Input: part model. Units: mm. Frame: model coordinates. Coordinates: 2 decimals unless noted, no trailing zeros. Loops run counter-clockwise (first coordinate to the right, second up) from the corner with the lowest first, then second, coordinate; pieces in that order, holes last.
Item 1: Section A-A on y = 128. Return loops of the section in (x, z), and give its area (3 significant figures).
Item 2: Ray query, line 1 along X through (y, z) = (164, -1.4); line 2 along Y through (x, z) = (-80, 0.85) (3 decimals); line 3 along Y through (x, z) = (14.5, -0.75) (3 decimals). Return the intervals inside material, ascending.
Item 3: Section C-C on z = -0.1. Give the number of separate pieces and of enclosed holes in the cut face, and give its area (3 significant figures).
```python
from build123d import *

# Parameters (mm, degrees)
SKETCH1_W                     = 382.775
SKETCH1_H                     = 238.275
BOSS_EXTRUDE1_DEPTH           = 1.5875
SKETCH3_W                     = 38.1
SKETCH3_H                     = 6.35
WELD_TABS_EXTRUDE_DEPTH       = 3.175
SKETCH4_R                     = 1.5875
WELD_TABS_TEAR_DROP_CUT_DEPTH = 3.175
WELD_TABS_CUTOUT_DEPTH        = 3.175


with BuildPart() as part:
    # Sketch1 → Boss-Extrude1 (new body, symmetric)
    with BuildSketch(Plane.XY):
        with Locations((-158.05, 122.3125)):
            Rectangle(SKETCH1_W, SKETCH1_H)
    extrude(amount=BOSS_EXTRUDE1_DEPTH, both=True)

    # Sketch3 → Weld Tabs Extrude (add)
    with BuildSketch(Plane.XY.offset(1.5875)):
        with Locations((-237.075, 0)):
            Rectangle(SKETCH3_W, SKETCH3_H)
        with Locations((-158.05, 0)):
            Rectangle(SKETCH3_W, SKETCH3_H)
        with Locations((-79.025, 0)):
            Rectangle(SKETCH3_W, SKETCH3_H)
    extrude(amount=-WELD_TABS_EXTRUDE_DEPTH)

    # Sketch4 → Weld Tabs Tear Drop Cut (cut)
    with BuildSketch(Plane.XY.offset(1.5875)):
        with Locations((-257.247532015, 2.052467985)):
            Circle(SKETCH4_R)
        with Locations((-216.902467985, 2.052467985)):
            Circle(SKETCH4_R)
        with Locations((-178.222532015, 2.052467985)):
            Circle(SKETCH4_R)
        with Locations((-137.877467985, 2.052467985)):
            Circle(SKETCH4_R)
        with Locations((-99.197532015, 2.052467985)):
            Circle(SKETCH4_R)
        with Locations((-58.852467985, 2.052467985)):
            Circle(SKETCH4_R)
    extrude(amount=-WELD_TABS_TEAR_DROP_CUT_DEPTH, mode=Mode.SUBTRACT)

    # Sketch6 → Weld Tabs Cutout (cut)
    with BuildSketch(Plane.XY.offset(1.5875)):
        with BuildLine():
            Line((-238.6625, 200.93125), (-238.6625, 162.83125))
            ThreePointArc((-238.6625, 162.83125), (-237.075, 161.24375), (-235.4875, 162.83125))
            Line((-235.4875, 162.83125), (-235.4875, 200.93125))
            ThreePointArc((-235.4875, 200.93125), (-237.075, 202.51875), (-238.6625, 200.93125))
        make_face()
        with BuildLine():
            Line((-317.6875, 200.93125), (-317.6875, 162.83125))
            ThreePointArc((-317.6875, 162.83125), (-316.1, 161.24375), (-314.5125, 162.83125))
            Line((-314.5125, 162.83125), (-314.5125, 200.93125))
            ThreePointArc((-314.5125, 200.93125), (-316.1, 202.51875), (-317.6875, 200.93125))
        make_face()
        with BuildLine():
            Line((-159.6375, 200.93125), (-159.6375, 162.83125))
            ThreePointArc((-159.6375, 162.83125), (-158.05, 161.24375), (-156.4625, 162.83125))
            Line((-156.4625, 162.83125), (-156.4625, 200.93125))
            ThreePointArc((-156.4625, 200.93125), (-158.05, 202.51875), (-159.6375, 200.93125))
        make_face()
        with BuildLine():
            Line((-80.6125, 200.93125), (-80.6125, 162.83125))
            ThreePointArc((-80.6125, 162.83125), (-79.025, 161.24375), (-77.4375, 162.83125))
            Line((-77.4375, 162.83125), (-77.4375, 200.93125))
            ThreePointArc((-77.4375, 200.93125), (-79.025, 202.51875), (-80.6125, 200.93125))
        make_face()
        with BuildLine():
            Line((-1.5875, 200.93125), (-1.5875, 162.83125))
            ThreePointArc((-1.5875, 162.83125), (0, 161.24375), (1.5875, 162.83125))
            Line((1.5875, 162.83125), (1.5875, 200.93125))
            ThreePointArc((1.5875, 200.93125), (0, 202.51875), (-1.5875, 200.93125))
        make_face()
        with BuildLine():
            Line((-238.6625, 141.3625), (-238.6625, 103.2625))
            ThreePointArc((-238.6625, 103.2625), (-237.075, 101.675), (-235.4875, 103.2625))
            Line((-235.4875, 103.2625), (-235.4875, 141.3625))
            ThreePointArc((-235.4875, 141.3625), (-237.075, 142.95), (-238.6625, 141.3625))
        make_face()
        with BuildLine():
            Line((-159.6375, 141.3625), (-159.6375, 103.2625))
            ThreePointArc((-159.6375, 103.2625), (-158.05, 101.675), (-156.4625, 103.2625))
            Line((-156.4625, 103.2625), (-156.4625, 141.3625))
            ThreePointArc((-156.4625, 141.3625), (-158.05, 142.95), (-159.6375, 141.3625))
        make_face()
        with BuildLine():
            Line((-80.6125, 141.3625), (-80.6125, 103.2625))
            ThreePointArc((-80.6125, 103.2625), (-79.025, 101.675), (-77.4375, 103.2625))
            Line((-77.4375, 103.2625), (-77.4375, 141.3625))
            ThreePointArc((-77.4375, 141.3625), (-79.025, 142.95), (-80.6125, 141.3625))
        make_face()
        with BuildLine():
            Line((-1.5875, 141.3625), (-1.5875, 103.2625))
            ThreePointArc((-1.5875, 103.2625), (0, 101.675), (1.5875, 103.2625))
            Line((1.5875, 103.2625), (1.5875, 141.3625))
            ThreePointArc((1.5875, 141.3625), (0, 142.95), (-1.5875, 141.3625))
        make_face()
        with BuildLine():
            Line((-238.6625, 81.79375), (-238.6625, 43.69375))
            ThreePointArc((-238.6625, 43.69375), (-237.075, 42.10625), (-235.4875, 43.69375))
            Line((-235.4875, 43.69375), (-235.4875, 81.79375))
            ThreePointArc((-235.4875, 81.79375), (-237.075, 83.38125), (-238.6625, 81.79375))
        make_face()
        with BuildLine():
            Line((-159.6375, 81.79375), (-159.6375, 43.69375))
            ThreePointArc((-159.6375, 43.69375), (-158.05, 42.10625), (-156.4625, 43.69375))
            Line((-156.4625, 43.69375), (-156.4625, 81.79375))
            ThreePointArc((-156.4625, 81.79375), (-158.05, 83.38125), (-159.6375, 81.79375))
        make_face()
        with BuildLine():
            Line((-80.6125, 81.79375), (-80.6125, 43.69375))
            ThreePointArc((-80.6125, 43.69375), (-79.025, 42.10625), (-77.4375, 43.69375))
            Line((-77.4375, 43.69375), (-77.4375, 81.79375))
            ThreePointArc((-77.4375, 81.79375), (-79.025, 83.38125), (-80.6125, 81.79375))
        make_face()
        with BuildLine():
            Line((-1.5875, 81.79375), (-1.5875, 43.69375))
            ThreePointArc((-1.5875, 43.69375), (0, 42.10625), (1.5875, 43.69375))
            Line((1.5875, 43.69375), (1.5875, 81.79375))
            ThreePointArc((1.5875, 81.79375), (0, 83.38125), (-1.5875, 81.79375))
        make_face()
        with BuildLine():
            Line((-317.6875, 141.3625), (-317.6875, 103.2625))
            ThreePointArc((-317.6875, 103.2625), (-316.1, 101.675), (-314.5125, 103.2625))
            Line((-314.5125, 103.2625), (-314.5125, 141.3625))
            ThreePointArc((-314.5125, 141.3625), (-316.1, 142.95), (-317.6875, 141.3625))
        make_face()
        with BuildLine():
            Line((-317.6875, 81.79375), (-317.6875, 43.69375))
            ThreePointArc((-317.6875, 43.69375), (-316.1, 42.10625), (-314.5125, 43.69375))
            Line((-314.5125, 43.69375), (-314.5125, 81.79375))
            ThreePointArc((-314.5125, 81.79375), (-316.1, 83.38125), (-317.6875, 81.79375))
        make_face()
    extrude(amount=-WELD_TABS_CUTOUT_DEPTH, mode=Mode.SUBTRACT)


solid = part.part
```
Results found:
1. outline: (-349.44, -1.59) - (-317.69, -1.59) - (-317.69, 1.59) - (-349.44, 1.59) - close; (-314.51, -1.59) - (-238.66, -1.59) - (-238.66, 1.59) - (-314.51, 1.59) - close; (-235.49, -1.59) - (-159.64, -1.59) - (-159.64, 1.59) - (-235.49, 1.59) - close; (-156.46, -1.59) - (-80.61, -1.59) - (-80.61, 1.59) - (-156.46, 1.59) - close; (-77.44, -1.59) - (-1.59, -1.59) - (-1.59, 1.59) - (-77.44, 1.59) - close; (1.59, -1.59) - (33.34, -1.59) - (33.34, 1.59) - (1.59, 1.59) - close
1. area: 1,160 mm2
2. line 1: x = -349.44 to -317.69, -314.51 to -238.66, -235.49 to -159.64, -156.46 to -80.61, -77.44 to -1.59, 1.59 to 33.34
2. line 2: y = -3.175 to 42.441, 83.047 to 102.01, 142.615 to 161.578, 202.184 to 241.45
2. line 3: y = 3.175 to 241.45
3. separate pieces: 1
3. enclosed holes: 15
3. area: 90,000 mm2
